from build123d import *

# Parameters (mm, degrees)
SALIENTE_EXTRUIR1_DEPTH = 50
CROQUIS2_R              = 2.5
CORTAR_EXTRUIR1_DEPTH   = 10
CROQUIS3_R              = 2.5
CORTAR_EXTRUIR2_DEPTH   = 10


with BuildPart() as part:
    # Croquis1 → Saliente-Extruir1 (new body)
    with BuildSketch(Plane(origin=(0, 0, 0), x_dir=(0, 0, -1), z_dir=(1, 0, 0))):
        Polygon((-20.239694924, -215.034421421), (-20.239694924, 41.965578579), (-18.239694924, 41.965578579), (-18.239694924, -213.034421421), (41.760305076, -213.034421421), (41.760305076, -215.034421421), align=None)
    extrude(amount=SALIENTE_EXTRUIR1_DEPTH)

    # Croquis2 → Cortar-Extruir1 (cut)
    with BuildSketch(Plane(origin=(0, -213.034421421, 0), x_dir=(1, 0, 0), z_dir=(0, 1, 0))):
        with Locations(Location((25, 11.760305076, 0), (0, 0, 270))):
            Circle(CROQUIS2_R)
    extrude(amount=-CORTAR_EXTRUIR1_DEPTH, mode=Mode.SUBTRACT)

    # Croquis3 → Cortar-Extruir2 (cut)
    with BuildSketch(Plane(origin=(0, 0, 18.239694924), x_dir=(-1, 0, 0), z_dir=(0, 0, -1))):
        with Locations(Location((-13.01, 19.730578579, 0), (0, 0, 90))):
            Circle(CROQUIS3_R)
    extrude(amount=-CORTAR_EXTRUIR2_DEPTH, mode=Mode.SUBTRACT)


solid = part.part
Can you work these out from the model? Positions are in its coordinate system, mm. A direction names the side the tool comes from. Round coordinates to 2 decimals unless told otherwise and drop trailing zeros. Order: outer loops, then holes, each group sorted by start corner. A loop starts at its lowest first (then second) coordinate and runs counter-clockwise, first axis right, second up. Notation, with made-up numbers: (-37.5, 32.5) - (12.5, 32.5) arc R30 ccw to (12.5, 61.5) - close; hole circle Ø7 at (70.5, 42.5). An arc over 180 degrees is marked (long way). Answer in a Markdown table with one row per item.
(1) Suppose I cut it at C-C, the plane y = -135. Please give me the cut outline in (x, z), plus the area to 3 significant figures.
From the geometry:
| item | result |
|---|---|
| outline | (0, 18.24) - (50, 18.24) - (50, 20.24) - (0, 20.24) - close |
| area | 100 mm2 |
(2) Suppose I cut it at A-A, the plane x = 13.01. Please give me the cut outline in (y, z).
From the geometry:
| item | result |
|---|---|
| outline | (-215.03, -41.76) - (-213.03, -41.76) - (-213.03, 18.24) - (17.23, 18.24) - (17.23, 20.24) - (-215.03, 20.24) - close; (22.23, 18.24) - (41.97, 18.24) - (41.97, 20.24) - (22.23, 20.24) - close |
(3) If we mould it in two halves opening along X, with no side actions, what happens to faces 3 (the face through (25, -84, 18.24)), 4 (the face through (50, -86, 19)), 5 (the face through (27.48, -214.02, -12.09))? For each: released by +X, released by -X, zero draft, split by the parting line, or undercut.
From the geometry:
| item | result |
|---|---|
| face 3 | zero draft |
| face 4 | released by +X |
| face 5 | undercut |
(4) For P1, Ø3, axis at x = 13.01, y = 19.73, coming from the -Z side; P2, Ø8, axis at x = 33.5, y = -65.5, coming from the -Z side, each with a flat end and sliding along its axis, tell me the tip position at first contact or that it passes through.
From the geometry:
| item | result |
|---|---|
| P1 | passes through |
| P2 | stops at z = 18.24 |
(5) Which directions (+Z, -Z, +X, -X, +Y, -Y) give clear straight access to the entire face, cutting with the end or side of a thin tool? Please do faces 1 (the face through (19, -213.034, -11)), 2 (the face through (25, -88, 20.24)).
From the geometry:
| item | result |
|---|---|
| face 1 | -Z, +X, -X, +Y |
| face 2 | +Z, +X, -X, +Y, -Y |
(6) Suppose I cut it at B-B, the plane z = 0. Please give me the cut outline in (x, y).
From the geometry:
| item | result |
|---|---|
| outline | (0, -215.03) - (50, -215.03) - (50, -213.03) - (0, -213.03) - close |
(7) Please list where these lines run through material, in increasing order: L1, parallel to Y at x = 24, z = -26; L2, parallel to Z at x = 24, y = -3. Write a range as from..to.
From the geometry:
| item | result |
|---|---|
| L1 | y = -215.03..-213.03 |
| L2 | z = 18.24..20.24 |
